```python
from build123d import *

# Parameters (mm, degrees)
F0_R     = 4.826
F1_DEPTH = 4.826


with BuildPart() as f1:
    # F0 (on Front) → F1 (new body)
    with BuildSketch(Plane.XZ):
        with BuildLine():
            Line((-6.199785, -15.992633), (6.499093, -16.161406))
            Line((6.499093, -16.161406), (6.199785, -11.344696))
            ThreePointArc((6.199785, -11.344696), (12.927958, -0.085905), (6.35, 11.261304))
            Line((6.35, 11.261304), (6.35, 16.087304))
            Line((6.35, 16.087304), (-6.35, 16.087304))
            Line((-6.35, 16.087304), (-6.35, 11.261304))
            ThreePointArc((-6.35, 11.261304), (-12.927958, 0.085905), (-6.499093, -11.175923))
            Line((-6.499093, -11.175923), (-6.199785, -15.992633))
        make_face()
        Circle(F0_R, mode=Mode.SUBTRACT)
    extrude(amount=F1_DEPTH)


solid = f1.part
```
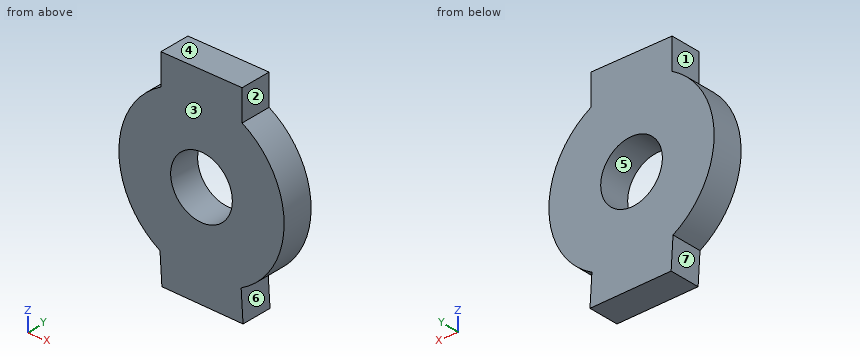
Here's how the part is built. I have some questions about the finished solid (model axes, mm). Face numbers are marked on the shaded views. A direction names the side the tool comes from. Round coordinates to 2 decimals unless told otherwise and drop trailing zeros. Loops run counter-clockwise (first coordinate to the right, second up) from the corner with the lowest first, then second, coordinate; pieces in that order, holes last. Notation, with made-up numbers: (57.5, -26) -> (106.5, -26) arc R20 ccw to (106.5, -4) -> close; hole circle Ø9 at (10.25, -14). An arc over 180 degrees is marked (long way). Answer as CSV lines item,"result". Start each with the question number.
1. Imagine slicing it at B-B on y = -1.7. Write out the boundary of the cut face in (x, z).
2. I need wall thicknesses on probe 1 along Z at (x, y) = (0.5, -0.3); probe 2 along X at (y, z) = (-1.6, 12); probe 3 along Z at (x, y) = (-1, -0.4). Which ranges of each line are inside material? Lowest first, please. Write a range as from..to.
3. I'm going to push flat-ended pins straight in: P1, Ø2, axis at x = -5, y = -4, coming from the -Z side; P2, Ø8.5, axis at x = 0, z = 0, coming from the +Y side; P3, Ø2, axis at y = -4, z = 12, coming from the +X side. Where does each tip first touch, or does it pass through?
4. Imagine slicing it at D-D on x = 8.25. Write out the boundary of the cut face in (y, z).
5. If we mould it in two halves opening along Z, with no side actions, what happens to the marked faces 4, 5, 6 and 7? For each: pulls with the +Z half, pulls with the -Z half, needs draft (parallel to the pull), parting line crosses it, or undercut.
6. For the marked faces 1, 2 and 3, which set-ups out of +Z, -Z, +X, -X, +Y, -Y let a thin tool reach every point of the face, with its end or its side?
7. Imagine slicing it at A-A on z = 0. Write out the boundary of the cut face in (x, y), plus the area to 3 significant figures.
8. Imagine slicing it at C-C on x = 0. Write out the boundary of the cut face in (y, z).
Solution:
1,outline,"(-6.5, -11.18) -> (-6.2, -15.99) -> (6.5, -16.16) -> (6.2, -11.34) arc R12.93 ccw to (6.35, 11.26) -> (6.35, 16.09) -> (-6.35, 16.09) -> (-6.35, 11.26) arc R12.93 ccw to start; hole circle Ø9.65 at (0, 0)"
2,probe 1,"-16.08..-4.8, 4.8..16.09"
2,probe 2,"-6.35..6.35"
2,probe 3,"-16.06..-4.72, 4.72..16.09"
3,P1,"z = -16.02"
3,P2,"through"
3,P3,"x = 6.79"
4,outline,"(-4.83, -9.95) -> (0, -9.95) -> (0, 9.95) -> (-4.83, 9.95) -> close"
5,face 4,"pulls with the +Z half"
5,face 5,"undercut"
5,face 6,"undercut"
5,face 7,"pulls with the -Z half"
6,face 1,"+Z, -X, +Y, -Y"
6,face 2,"+Z, +X, +Y, -Y"
6,face 3,"+Z, -Z, +X, -X, -Y"
7,outline,"(-12.93, -4.83) -> (-4.83, -4.83) -> (-4.83, 0) -> (-12.93, 0) -> close; (4.83, -4.83) -> (12.93, -4.83) -> (12.93, 0) -> (4.83, 0) -> close"
7,area,"78.2 mm²"
8,outline,"(-4.83, -16.08) -> (0, -16.08) -> (0, -4.83) -> (-4.83, -4.83) -> close; (-4.83, 4.83) -> (0, 4.83) -> (0, 16.09) -> (-4.83, 16.09) -> close"
